Study the drawing (mm; zero at the part's minimum x, y, z) and answer. Coordinates: 2 decimals unless noted, no trailing zeros. Write each loop counter-clockwise with the first axis right and the second up, starting at its lowest first coordinate (ties: lowest second). Pieces come first, ordered by that corner, then holes. Notation, with made-up numbers: (0.25, 1) -> (42.25, 1) arc R12 cw to (42.25, 22) -> close; hole circle Ø1 at (65.25, 11.5). An arc over 180 degrees is marked (long way). Write item = value, one per line. Start each with the question number.
1) Flat-ended cylindrical pins translate along their axes: pin 1 Ø5 at (x, y) = (5.4, 8.19) entering from +Z (3 decimals); pin 2 Ø1.5 at (x, z) = (13, 2) entering from -Y. Find the tip coordinate at first contact, or state that the pin passes through.
2) For a pull along Y with two mould halves and no side action, classify the marked faces 1, 2, 3 and 4 as released by +Y, released by -Y, zero draft, split by the parting line, or undercut.
3) Section A-A (y = 19.62) is taken. Determine the outline of the cut face in (x, z) (1 decimal).
4) Find the intervals of material crossed by line 1 along Y through (x, z) = (12, 2.45) (1 decimal); line 2 along X through (y, z) = (7, 2.8); line 3 along Y through (x, z) = (13.5, 2.25) (1 decimal), in increasing order. Write a range as from..to.
5) Section C-C (z = 1.25) is taken. Count the separate pieces of the cut face and the enclosed holes in it, plus the area to 3 significant figures.
6) Section B-B (y = 8.19) is taken. Determine the outline of the cut face in (x, z) (1 decimal).
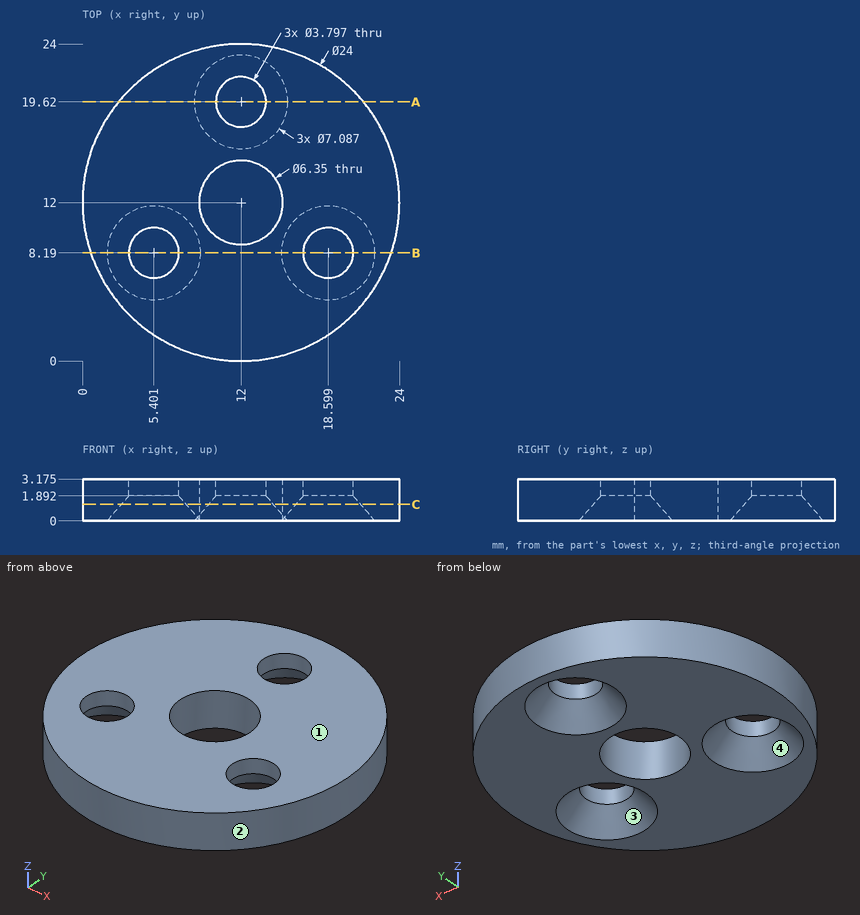
Answer key:
q1.pin_1 = 3.175
q1.pin_2 = 0
q2.face_1 = zero draft
q2.face_2 = split by the parting line
q2.face_3 = undercut
q2.face_4 = undercut
q3.outline = (2.7, 0) -> (8.5, 0) -> (10.1, 1.9) -> (10.1, 3.2) -> (2.7, 3.2) -> close; (13.9, 1.9) -> (15.5, 0) -> (21.3, 0) -> (21.3, 3.2) -> (13.9, 3.2) -> close
q4.line_1 = 0..8.8, 15.2..17.7, 21.5..24
q4.line_2 = 1.09..3.92, 6.88..17.12, 20.08..22.91
q4.line_3 = 0.1..9.2, 14.8..18.5, 20.8..23.9
q5.separate_pieces = 1
q5.enclosed_holes = 4
q5.area = 364 mm^2
q6.outline = (0.6, 0) -> (1.9, 0) -> (3.5, 1.9) -> (3.5, 3.2) -> (0.6, 3.2) -> close; (7.3, 1.9) -> (8.9, 0) -> (15.1, 0) -> (16.7, 1.9) -> (16.7, 3.2) -> (7.3, 3.2) -> close; (20.5, 1.9) -> (22.1, 0) -> (23.4, 0) -> (23.4, 3.2) -> (20.5, 3.2) -> close
